from build123d import *

# Parameters (mm, degrees)
BOSS_EXTRUDE1_DEPTH = 15
SKETCH2_W           = 10
SKETCH2_H           = 5
BOSS_EXTRUDE2_DEPTH = 130
FILLET3_R           = 1
FILLET4_R           = 1
FILLET5_R           = 1
FILLET6_R           = 1
CUT_EXTRUDE1_REACH  = 132.54
SKETCH3_R           = 2.5
SKETCH3_R_2         = 1.5


with BuildPart() as part:
    # Sketch1 → Boss-Extrude1 (new body)
    with BuildSketch(Plane.XY):
        Polygon((-5.618855965, 9), (-5.618855965, 0), (6.381144035, 0), (6.381144035, 9), (4.381144035, 9), (4.381144035, 7), (5.399108107, 7), (5.399108107, 2), (-4.600891893, 2), (-4.600891893, 7), (-3.600891893, 7), (-3.600891893, 9), align=None)
    extrude(amount=BOSS_EXTRUDE1_DEPTH)

    # Sketch2 → Boss-Extrude2 (add)
    with BuildSketch(Plane.XZ):
        with Locations((0.381144035, 7.5)):
            Rectangle(SKETCH2_W, SKETCH2_H)
    extrude(amount=BOSS_EXTRUDE2_DEPTH)

    # Fillet3
    fillet3_edges = [part.edges().sort_by_distance(p)[0] for p in [
        (0.381144035, 0, 10),
        (-4.618855965, 0, 7.5),
    ]]
    fillet(fillet3_edges, radius=FILLET3_R - 0.0001)  # a hair under: the kernel refuses the full size

    # Fillet4
    fillet4_edges = [part.edges().sort_by_distance(p)[0] for p in [
        (-0.118805965, 0, 5),
    ]]
    fillet(fillet4_edges, radius=FILLET4_R - 0.0001)  # a hair under: the kernel refuses the full size

    # Fillet5
    fillet5_edges = [part.edges().sort_by_distance(p)[0] for p in [
        (5.381144035, 0, 7.5),
    ]]
    fillet(fillet5_edges, radius=FILLET5_R - 0.0001)  # a hair under: the kernel refuses the full size

    # Fillet6
    fillet6_edges = [part.edges().sort_by_distance(p)[0] for p in [
        (-4.618855965, -130, 7.5),
        (0.381144035, -130, 5),
        (0.381144035, -130, 10),
        (5.381144035, -130, 7.5),
    ]]
    fillet(fillet6_edges, radius=FILLET6_R)

    # Sketch3 → Cut-Extrude1 (cut, up to next)
    with BuildSketch(Plane(origin=(0, 0, 5), x_dir=(-1, 0, 0), z_dir=(0, 0, -1)), mode=Mode.PRIVATE) as cut_extrude1_sk1:
        with Locations((0, -11)):
            Circle(SKETCH3_R)
    cut_extrude1_tool1 = extrude(cut_extrude1_sk1.sketch, amount=-CUT_EXTRUDE1_REACH, mode=Mode.PRIVATE) & part.part
    # Sketch3 → Cut-Extrude1 (cut, up to next)
    with BuildSketch(Plane(origin=(0, 0, 5), x_dir=(-1, 0, 0), z_dir=(0, 0, -1)), mode=Mode.PRIVATE) as cut_extrude1_sk2:
        with Locations((0, -124)):
            Circle(SKETCH3_R_2)
    cut_extrude1_tool2 = extrude(cut_extrude1_sk2.sketch, amount=-CUT_EXTRUDE1_REACH, mode=Mode.PRIVATE) & part.part
    # Sketch3 → Cut-Extrude1 (cut, up to next)
    with BuildSketch(Plane(origin=(0, 0, 5), x_dir=(-1, 0, 0), z_dir=(0, 0, -1)), mode=Mode.PRIVATE) as cut_extrude1_sk3:
        with Locations((0, -76)):
            Circle(SKETCH3_R_2)
    cut_extrude1_tool3 = extrude(cut_extrude1_sk3.sketch, amount=-CUT_EXTRUDE1_REACH, mode=Mode.PRIVATE) & part.part
    add(cut_extrude1_tool1.solids().sort_by_distance((0, -11, 5))[0], mode=Mode.SUBTRACT)
    add(cut_extrude1_tool2.solids().sort_by_distance((0, -124, 5))[0], mode=Mode.SUBTRACT)
    add(cut_extrude1_tool3.solids().sort_by_distance((0, -76, 5))[0], mode=Mode.SUBTRACT)


solid = part.part
Build history of the part. All positions in model axes, mm. A direction names the side the tool comes from. Coordinates: 2 decimals unless noted, no trailing zeros. Write each loop counter-clockwise with the first axis right and the second up, starting at its lowest first coordinate (ties: lowest second). Pieces come first, ordered by that corner, then holes.
(1) Pin check, flat tips, straight feed: pin 1 Ø0.5 at (x, z) = (5, 10) entering from -Y; pin 2 Ø1 at (y, z) = (-47, 5.5) entering from -X; pin 3 Ø5 at (x, y) = (-0.5, -106.5) entering from -Z; pin 4 Ø1.1 at (x, z) = (-4, 7.5) entering from -Y. Stop position of each tip, or through.
(2) Mould opens along Y. For faces 1 (the flat face through (5.399, 5, 7)), 2 (the flat face through (0, 0, 2)), 3 (the cylindrical face through (-0.806, -74.735, 7.465)), 4 (the flat face through (5.381, -64, 7)) say: pulls with the +Y half, pulls with the -Y half, needs draft (parallel to the pull), parting line crosses it, or undercut.
(3) Cut at B-B on z = 7.75. State how many separate pieces and enclosed holes the cut face has, and give its area (3 significant figures).
(4) 3-axis set-ups, long thin cutter, end or side, ignore diameter. For faces 5 (the flat face through (-4.619, -64, 7)), 6 (the flat face through (0, -64, 5)), 7 (the flat face through (-4.601, 4, 7)): which of +Z, -Z, +X, -X, +Y, -Y reach the whole face in a straight line?
(5) Cut at C-C on z = 1.25. List the corners of the cut face in (x, y).
(6) Cut at D-D on y = -11. List the corners of the cut face in (x, z), and give its area (3 significant figures).
(7) Cut at A-A on y = -124. List the corners of the cut face in (x, z), and give its area (3 significant figures).
(8) Drill centre lines: line 1 (Y direction, x = 0, z = 6.2); line 2 (X direction, y = -124, z = 7.3); line 3 (X direction, y = 3, z = 4.25). Where is each one in solid material? Low to high.
Working result:
1. pin 1: stops at y = -129.66
1. pin 2: stops at x = -4.62
1. pin 3: stops at z = 5
1. pin 4: stops at y = -130
2. face 1: undercut
2. face 2: pulls with the -Y half
2. face 3: undercut
2. face 4: needs draft
3. separate pieces: 1
3. enclosed holes: 3
3. area: 1,310 mm2
4. face 5: +Z, -Z, -X, -Y
4. face 6: -Z, +X, -X, -Y
4. face 7: +Z, -Z
5. outline: (-5.62, 0) - (6.38, 0) - (6.38, 9) - (4.38, 9) - (4.38, 7) - (5.4, 7) - (5.4, 2) - (-4.6, 2) - (-4.6, 7) - (-3.6, 7) - (-3.6, 9) - (-5.62, 9) - close
6. outline: (-4.62, 5) - (-2.5, 5) - (-2.5, 10) - (-4.62, 10) - close; (2.5, 5) - (5.38, 5) - (5.38, 10) - (2.5, 10) - close
6. area: 25.0 mm2
7. outline: (-4.62, 5) - (-1.5, 5) - (-1.5, 10) - (-4.62, 10) - close; (1.5, 5) - (5.38, 5) - (5.38, 10) - (1.5, 10) - close
7. area: 35.0 mm2
8. line 1: y = -130 to -125.5, -122.5 to -77.5, -74.5 to -13.5, -8.5 to 2
8. line 2: x = -4.62 to -1.5, 1.5 to 5.38
8. line 3: x = -5.62 to -4.6, 5.4 to 6.38
